from build123d import *

# Parameters (mm, degrees)
SKETCH1_R           = 1.27
SKETCH1_R_2         = 3.81
SKETCH1_W           = 9.271
SKETCH1_H           = 9.271
BOSS_EXTRUDE1_DEPTH = 2.54


with BuildPart() as part:
    # Sketch1 → Boss-Extrude1 (new body)
    with BuildSketch(Plane(origin=(0, 0, 0), x_dir=(1, 0, 0), z_dir=(0, 1, 0))):
        with BuildLine():
            Line((48.26, 0), (-48.26, 0))
            ThreePointArc((-48.26, 0), (-53.138298297, 8.070705976), (-47.844237094, 15.875))
            Line((-47.844237094, 15.875), (-22.444237094, 15.875))
            Line((-22.444237094, 15.875), (-8.5852, 25.4))
            Line((-8.5852, 25.4), (8.5852, 25.4))
            Line((8.5852, 25.4), (22.444237094, 15.875))
            Line((22.444237094, 15.875), (47.844237094, 15.875))
            ThreePointArc((47.844237094, 15.875), (53.138298297, 8.070705976), (48.26, 0))
        make_face()
        with Locations(Location((-8.5852, 16.7767, 0), (0, 0, 270))):
            Circle(SKETCH1_R, mode=Mode.SUBTRACT)
        with Locations(Location((8.5852, 16.7767, 0), (0, 0, 90))):
            Circle(SKETCH1_R, mode=Mode.SUBTRACT)
        with Locations(Location((-44.401571021, 7.841892929, 0), (0, 0, 270))):
            Circle(SKETCH1_R_2, mode=Mode.SUBTRACT)
        with Locations(Location((44.401571021, 7.841892929, 0), (0, 0, 90))):
            Circle(SKETCH1_R_2, mode=Mode.SUBTRACT)
        with Locations((0, 16.7767)):
            Rectangle(SKETCH1_W, SKETCH1_H, mode=Mode.SUBTRACT)
    extrude(amount=BOSS_EXTRUDE1_DEPTH)


solid = part.part
Source: CAD feature listing. Evaluate the final solid. Frame: model axes, mm. A direction names the side the tool comes from. Coordinates: 2 decimals unless noted, no trailing zeros. Order: outer loops, then holes, each group sorted by start corner. A loop starts at its lowest first (then second) coordinate and runs counter-clockwise, first axis right, second up. Notation, with made-up numbers: M 88,89 L 94,89 A31 ccw 94,113 Z; hole C 27,15 d11. An arc over 180 degrees is marked long. Write each question's results on one line, items separated by ' | '. Start each with the question number.
1. Section C-C, the plane z = -19.75. Return the cut outline in (x, y).
2. Draft query along X for faces 5 (the face through (1, 0, -10)), 6 (the face through (53.134, 1.252, -8.21)), 7 (the face through (-4.636, 1, -17)). Return one class per face: +X half, -X half, draft (parallel to the pull), parting line (faces both ways), or undercut.
3. Material intervals for L1, parallel to X at y = 2.25, z = -6.25; L2, parallel to X at y = 1.6, z = -15.75; L3, parallel to X at y = 1.65, z = -16.75, sorted ascending.
4. Reachability of faces 1 (the face through (0, 1, -21.412)), 2 (the face through (35, 1, -15.875)), 3 (the face through (-53.14, 1.25, -7.93)), 4 (the face through (-35, 1, -15.875)) from +Z, -Z, +X, -X, +Y, -Y: full face, straight path, thin tool, end or side. Return the list, or none.
5. Pin query (flat end, axial travel): pin 1 (1.5 mm diameter, centred on x = 38.5, y = 2, fed in from -Z) (3 decimals); pin 2 (2 mm diameter, centred on x = 8.59, z = -16.78, fed in from -Y). Return the tip coordinate at first contact, or that it passes through.
6. Section D-D, the plane x = 38.5. Return the cut outline in (y, z) (3 decimals).
7. Section A-A, the plane z = -10.75. Return the cut outline in (x, y), then the cut area to 3 significant figures.
8. Section B-B, the plane y = 1.1. Return the cut outline in (x, z) (1 decimal).
Solution:
1) outline: M -16.81,0 L -4.64,0 L -4.64,2.54 L -16.81,2.54 Z; M 4.64,0 L 16.81,0 L 16.81,2.54 L 4.64,2.54 Z
2) face 5: draft | face 6: +X half | face 7: undercut
3) L1: -53 to -47.86, -40.94 to 40.94, 47.86 to 53 | L2: -48.12 to -9.33, -7.84 to -4.64, 4.64 to 7.84, 9.33 to 48.12 | L3: -21.17 to -9.85, -7.32 to -4.64, 4.64 to 7.32, 9.85 to 21.17
4) face 1: +Y, -Y | face 2: -Z, +X, +Y, -Y | face 3: -X, +Y, -Y | face 4: -Z, -X, +Y, -Y
5) pin 1: z = -15.875 | pin 2: through
6) outline: M 0,-15.875 L 2.54,-15.875 L 2.54,0 L 0,0 Z
7) outline: M -52.64,0 L -46.86,0 L -46.86,2.54 L -52.64,2.54 Z; M -41.94,0 L 41.94,0 L 41.94,2.54 L -41.94,2.54 Z; M 46.86,0 L 52.64,0 L 52.64,2.54 L 46.86,2.54 Z | area: 242 mm²
8) outline: M -48.3,0 A8.7 ccw -47.8,-15.9 L -22.4,-15.9 L -8.6,-25.4 L 8.6,-25.4 L 22.4,-15.9 L 47.8,-15.9 A8.7 ccw 48.3,0 Z; hole C -44.4,-7.8 d7.6; hole C -8.6,-16.8 d2.5; hole M -4.6,-21.4 L 4.6,-21.4 L 4.6,-12.1 L -4.6,-12.1 Z; hole C 8.6,-16.8 d2.5; hole C 44.4,-7.8 d7.6
